from build123d import *

# Parameters (mm, degrees)
SKETCH_1_W      = 24
SKETCH_1_H      = 24
EXTRUDE_5_DEPTH = 12
SHELL_2_T       = -1.95
SKETCH_5_W      = 17
SKETCH_5_H      = 17
EXTRUDE_6_DEPTH = 10


with BuildPart() as part:
    # ｽｹｯﾁ1 → ﾎﾞｽ - 押し出し5 (new body)
    with BuildSketch(Plane.XY):
        with Locations((12, 12)):
            Rectangle(SKETCH_1_W, SKETCH_1_H)
    extrude(amount=EXTRUDE_5_DEPTH)

    # ｼｪﾙ2
    shell_2_openings = [part.faces().sort_by_distance(p)[0] for p in [
        (12, 12, 12),
    ]]
    offset(amount=SHELL_2_T, openings=shell_2_openings, kind=Kind.INTERSECTION)

    # ｽｹｯﾁ5 → ﾎﾞｽ - 押し出し6 (add)
    with BuildSketch(Plane.XY.offset(1.95)):
        with Locations((12, 12)):
            Rectangle(SKETCH_5_W, SKETCH_5_H)
    extrude(amount=EXTRUDE_6_DEPTH)


solid = part.part
Work out the finished part from the listing and answer in its coordinate system (mm). A direction names the side the tool comes from. Give positions to 0.01 mm unless a question says otherwise; leave off trailing zeros. Order: outer loops, then holes, each group sorted by start corner. A loop starts at its lowest first (then second) coordinate and runs counter-clockwise, first axis right, second up. Notation, with made-up numbers: M 81,39.5 L 92,39.5 A22 ccw 92,76.5 Z; hole C 3.25,84 d4. An arc over 180 degrees is marked long. Return JSON: item names as keys, results as strings.
Q1. Find section B-B, the plane y = 17. Write down the section's boundary in (x, z), and give its area (3 significant figures).
Answer below:
{"outline": "M 0,0 L 24,0 L 24,12 L 22.05,12 L 22.05,1.95 L 20.5,1.95 L 20.5,11.95 L 3.5,11.95 L 3.5,1.95 L 1.95,1.95 L 1.95,12 L 0,12 Z", "area": "256 mm^2"}
Q2. Which of the six approach directions +Z, -Z, +X, -X, +Y, -Y give full straight-line access (tool end or side, diameter ignored) to faces 4 (the face through (1.95, 12, 7)), 5 (the face through (12, 24, 6))?
Answer below:
{"face 4": "+Z", "face 5": "+Z, -Z, +X, -X, +Y"}
Q3. The mould has two halves that part along Y. Classify faces 1 (the face through (12, 0, 6)), 2 (the face through (0, 12, 6)), 3 (the face through (12, 22.05, 7)): pulls with the +Y half, pulls with the -Y half, needs draft (parallel to the pull), parting line crosses it, or undercut.
Answer below:
{"face 1": "pulls with the -Y half", "face 2": "needs draft", "face 3": "undercut"}
Q4. This flat-tipped pin is pushed along its axis until it touches: pin 1 (6 mm diameter, centred on x = 7, y = 10, fed in from +Z). Where does it stop, or does it pass through?
Answer below:
{"pin 1": "stops at z = 11.95"}
Q5. Find section D-D, the plane y = 2.5. Write down the section's boundary in (x, z), and give its area (3 significant figures).
Answer below:
{"outline": "M 0,0 L 24,0 L 24,12 L 22.05,12 L 22.05,1.95 L 1.95,1.95 L 1.95,12 L 0,12 Z", "area": "86.0 mm^2"}
Q6. Find the intervals of material crossed by line 1 along X through (y, z) = (18.5, 3.5); line 2 along Y through (x, z) = (2.25, 8.25), in increasing order. Write a range as [from, to].
Answer below:
{"line 1": "x = [0, 1.95], [3.5, 20.5], [22.05, 24]", "line 2": "y = [0, 1.95], [22.05, 24]"}
Q7. Find section A-A, the plane z = 5.5. Write down the section's boundary in (x, y).
Answer below:
{"outline": "M 0,0 L 24,0 L 24,24 L 0,24 Z; M 3.5,3.5 L 20.5,3.5 L 20.5,20.5 L 3.5,20.5 Z; hole M 1.95,1.95 L 22.05,1.95 L 22.05,22.05 L 1.95,22.05 Z"}
